Verification items for the finished model (mm, model axes). A direction names the side the tool comes from. Coordinates: 2 decimals unless noted, no trailing zeros. Order: outer loops, then holes, each group sorted by start corner. A loop starts at its lowest first (then second) coordinate and runs counter-clockwise, first axis right, second up. Notation, with made-up numbers: M -21.75,48 L 14.25,48 A20 ccw 14.25,72 Z; hole C -17.75,39 d6. An arc over 180 degrees is marked long. Write item = value, one per line.
```python
from build123d import *

# Parameters (mm, degrees)
F1_DEPTH = 80
F2_R     = 2
F3_DEPTH = 25


with BuildPart() as f1:
    # F0 (on Top) → F1 (new body)
    with BuildSketch(Plane.XY):
        Polygon((12, -4), (12, 4), (-12, 4), (-12, -4), (-2, -4), (-2, 2), (2, 2), (2, -4), align=None)
    extrude(amount=F1_DEPTH)

    # F2 (on face) → F3 (cut)
    with BuildSketch(Plane(origin=(0, 4, 0), x_dir=(-1, 0, 0), z_dir=(0, 1, 0))):
        with Locations((-8, 8)):
            Circle(F2_R)
        with Locations((-8, 24)):
            Circle(F2_R)
        with Locations((-8, 40)):
            Circle(F2_R)
        with Locations((-8, 56)):
            Circle(F2_R)
        with Locations((-8, 72)):
            Circle(F2_R)
        with Locations((8, 8)):
            Circle(F2_R)
        with Locations((8, 24)):
            Circle(F2_R)
        with Locations((8, 40)):
            Circle(F2_R)
        with Locations((8, 56)):
            Circle(F2_R)
        with Locations((8, 72)):
            Circle(F2_R)
        with Locations((-8, 88)):
            Circle(F2_R)
        with Locations((-8, 104)):
            Circle(F2_R)
        with Locations((-8, 120)):
            Circle(F2_R)
        with Locations((-8, 136)):
            Circle(F2_R)
        with Locations((-8, 152)):
            Circle(F2_R)
        with Locations((8, 88)):
            Circle(F2_R)
        with Locations((8, 104)):
            Circle(F2_R)
        with Locations((8, 120)):
            Circle(F2_R)
        with Locations((8, 136)):
            Circle(F2_R)
        with Locations((8, 152)):
            Circle(F2_R)
    extrude(amount=-F3_DEPTH, mode=Mode.SUBTRACT)


solid = f1.part
```
Item 1: Sectioned sample at B-B, the plane z = 56. Enter the section's corners in (x, y), then the cut area to 3 significant figures.
Report:
outline = M -12,-4 L -10,-4 L -10,4 L -12,4 Z; M -6,-4 L -2,-4 L -2,2 L 2,2 L 2,-4 L 6,-4 L 6,4 L -6,4 Z; M 10,-4 L 12,-4 L 12,4 L 10,4 Z
area = 104 mm^2
Item 2: Release check for a two-part mould opening along Z. For faces 1 (the flat face through (-12, 0, 39)), 2 (the flat face through (0, 3, 80)), 3 (the cylindrical face through (-6.526, 0.056, 9.352)) record: pulls with the +Z half, pulls with the -Z half, needs draft (parallel to the pull), parting line crosses it, or undercut.
Report:
face_1 = needs draft
face_2 = pulls with the +Z half
face_3 = undercut
Item 3: Scan lines: L1, parallel to Z at x = -8, y = -0.25; L2, parallel to Z at x = 8.75, y = 3.5; L3, parallel to X at y = -0.75, z = 69. Record each from-to range of solid material in increasing order. Write a range as from..to.
Report:
L1 = 0..6, 10..22, 26..38, 42..54, 58..70, 74..80
L2 = 0..6.15, 9.85..22.15, 25.85..38.15, 41.85..54.15, 57.85..70.15, 73.85..80
L3 = -12..-2, 2..12
Item 4: Sectioned sample at C-C, the plane x = -8. Enter the section's corners in (y, z).
Report:
outline = M -4,0 L 4,0 L 4,6 L -4,6 Z; M -4,10 L 4,10 L 4,22 L -4,22 Z; M -4,26 L 4,26 L 4,38 L -4,38 Z; M -4,42 L 4,42 L 4,54 L -4,54 Z; M -4,58 L 4,58 L 4,70 L -4,70 Z; M -4,74 L 4,74 L 4,80 L -4,80 Z
Item 5: Sectioned sample at A-A, the plane y = 1.25. Give the number of separate pieces and of enclosed holes in the cut face, then the cut area to 3 significant figures.
Report:
separate_pieces = 2
enclosed_holes = 10
area = 1,470 mm^2
Item 6: Tool access check on faces 4 (the cylindrical face through (9.6, 0.1, 22.8)), 5 (the flat face through (0, 2, 39)). Record the directions out of +Z, -Z, +X, -X, +Y, -Y that give a thin tool (end or side, any length) a straight path to the whole face; none if there is none.
Report:
face_4 = +Y, -Y
face_5 = +Z, -Z, -Y
Item 7: Gauge pin test, flat end, axial feed: pin 1 (1 mm diameter, centred on x = -3.5, y = 2.5, fed in from -Z). Record the tip position at first contact, or that the pin passes through.
Report:
pin_1 = 0
Item 8: Sectioned sample at D-D, the plane z = 64. Enter the section's corners in (x, y), then the cut area to 3 significant figures.
Report:
outline = M -12,-4 L -2,-4 L -2,2 L 2,2 L 2,-4 L 12,-4 L 12,4 L -12,4 Z
area = 168 mm^2
